Can you work these out from the model? Positions are in its coordinate system, mm. Face numbers are marked on the shaded views. A direction names the side the tool comes from. Give positions to 0.01 mm unless a question says otherwise; leave off trailing zeros. Write each loop counter-clockwise with the first axis right and the second up, starting at its lowest first coordinate (ties: lowest second). Pieces come first, ordered by that corner, then holes. Notation, with made-up numbers: (-10.5, -21.5) - (30.5, -21.5) arc R33 cw to (30.5, 9.5) - close; hole circle Ø8 at (10, 53). An arc over 180 degrees is marked (long way). Use a Markdown table: item, result. Add a question column.
```python
from build123d import *

# Parameters (mm, degrees)
SKETCH1_R           = 10
BOSS_EXTRUDE1_DEPTH = 20
BOSS_EXTRUDE1_TAPER = 3
SKETCH2_R           = 5
CUT_EXTRUDE1_DEPTH  = 4
CUT_EXTRUDE2_DEPTH  = 12
CHAMFER1_SIZE       = 1
CHAMFER1_SIZE2      = 0.577350269


with BuildPart() as part:
    # Sketch1 → Boss-Extrude1 (new body)
    with BuildSketch(Plane(origin=(0, 0, 0), x_dir=(1, 0, 0), z_dir=(0, 1, 0))):
        Circle(SKETCH1_R)
    extrude(amount=BOSS_EXTRUDE1_DEPTH, taper=BOSS_EXTRUDE1_TAPER)

    # Sketch2 → Cut-Extrude1 (cut)
    with BuildSketch(Plane.XZ):
        with Locations(Location((0, 0, 0), (0, 0, 270))):
            Circle(SKETCH2_R)
    extrude(amount=-CUT_EXTRUDE1_DEPTH, mode=Mode.SUBTRACT)

    # Sketch3 → Cut-Extrude2 (cut)
    with BuildSketch(Plane.XZ.offset(-4)):
        with BuildLine():
            Line((-1.732055507, -2.57098886), (3.04828024, -0.563903873))
            ThreePointArc((3.04828024, -0.563903873), (-1.200087257, 2.858284551), (-1.732055507, -2.57098886))
        make_face()
    extrude(amount=-CUT_EXTRUDE2_DEPTH, mode=Mode.SUBTRACT)

    # Chamfer1
    chamfer1_edges = [part.edges().sort_by_distance(p)[0] for p in [
        (0, 0, 5),
    ]]
    chamfer1_side = [part.faces().sort_by_distance(p)[0] for p in [
        (0, 2, 5),
    ]]
    chamfer(chamfer1_edges, length=CHAMFER1_SIZE, length2=CHAMFER1_SIZE2, reference=chamfer1_side[0])


solid = part.part
```
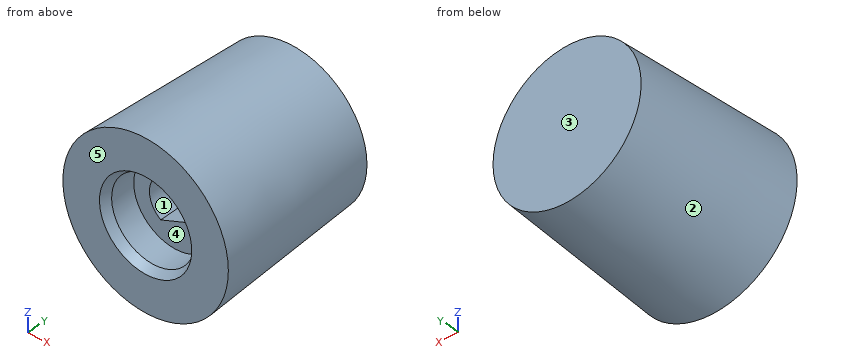
Q1. Suppose I cut it at A-A (y = 2). Please give me the cut outline in (x, z), and give its area (3 significant figures).
Q2. Suppose I cut it at B-B (x = 0). Please give me the cut outline in (y, z).
Q3. Suppose I cut it at C-C (y = 16.5). Please give me the cut outline in (x, z).
Q4. If I drill on probe 1 along Y at (x, z) = (-3.25, 2); probe 2 along Z at (x, y) = (0, 10.5); probe 3 along X at (y, z) = (8.5, 1.5), over which ranges is the centre line in solid material (lowest first)? Write a range as [from, to].
Q5. Suppose I cut it at D-D (y = 5.5). Please give me the cut outline in (x, z), and give its area (3 significant figures).
Q6. I'm going to push flat-ended pins straight in: P1, Ø4.5, axis at x = 0, z = 1.5, coming from the -Y side; P2, Ø1, axis at y = 14.5, z = 6, coming from the +X side; P3, Ø6, axis at x = 4.5, y = 15, coming from the +Z side. Where does each tip first touch, or does it pass through?
Q7. If we mould it in two halves opening along X, with no side actions, what happens to the marked faces 1, 2 and 3? For each: released by +X, released by -X, zero draft, split by the parting line, or undercut.
Q8. On a 3-axis mill with a long thin cutter (end or side, diameter ignored), from which of +Z, -Z, +X, -X, +Y, -Y can I reach the whole of each face in a straight line? I mean the marked faces 4 and 5. Say none if no direction works.
Derived:
| question | item | result |
|---|---|---|
| 1 | outline | circle Ø19.79 at (0, 0); hole circle Ø10 at (0, 0) |
| 1 | area | 229 mm² |
| 2 | outline | (0, -10) - (20, -8.95) - (20, 8.95) - (0, 10) - (0, 5.58) - (1, 5) - (4, 5) - (4, 3.1) - (16, 3.1) - (16, -1.84) - (4, -1.84) - (4, -5) - (1, -5) - (0, -5.58) - close |
| 3 | outline | circle Ø18.27 at (0, 0) |
| 4 | probe 1 | [4, 20] |
| 4 | probe 2 | [-9.45, -1.84], [3.1, 9.45] |
| 4 | probe 3 | [-9.44, -2.71], [2.71, 9.44] |
| 5 | outline | circle Ø19.42 at (0, 0); hole (-1.73, -2.57) - (3.05, -0.56) arc R3.1 ccw (long way) to start |
| 5 | area | 271 mm² |
| 6 | P1 | y = 4 |
| 6 | P2 | x = 7.43 |
| 6 | P3 | z = 9.12 |
| 7 | face 1 | undercut |
| 7 | face 2 | split by the parting line |
| 7 | face 3 | zero draft |
| 8 | face 4 | -Y |
| 8 | face 5 | +Z, -Z, +X, -X, -Y |
